Could you check a few things on this drawing? It's one solid part, dimensions in mm from its lowest x, y, z. A direction names the side the tool comes from. Give positions to 0.01 mm unless a question says otherwise; leave off trailing zeros. Loops run counter-clockwise (first coordinate to the right, second up) from the corner with the lowest first, then second, coordinate; pieces in that order, holes last. Notation, with made-up numbers: M -23,-17.75 L 28,-17.75 A30 cw 28,10.25 Z; hole C -36,72.5 d8. An arc over 180 degrees is marked long. Return JSON: item names as keys, results as strings. Group by question number.
1. If we section it at D-D (x = 144): Write out the boundary of the cut face in (y, z), plus the area to 3 significant figures.
2. Please list where these lines run through material, in increasing order: line 1 (X direction, y = 18.5, z = 7); line 2 (Y direction, x = 80.5, z = 52); line 3 (Z direction, x = 131, y = 30.5).
3. If we section it at B-B (y = 16.5): Write out the boundary of the cut face in (x, z) (1 decimal), plus the area to 3 significant figures.
4. For pin 1 (12 mm diameter, centred on x = 52.5, y = 52.5, fed in from -Z); pin 2 (4 mm diameter, centred on x = 97, y = 59.5, fed in from +Z); pin 3 (4 mm diameter, centred on x = 50.5, y = 47.5, fed in from -Z), each with a flat end and sliding along its axis, tell me the tip position at first contact or that it passes through.
5. For the marked faces 1, 2 and 3, which set-ups out of +Z, -Z, +X, -X, +Y, -Y let a thin tool reach every point of the face, with its end or its side?
6. If we section it at C-C (x = 47): Write out the boundary of the cut face in (y, z).
7. If we section it at A-A (z = 51.5): Write out the boundary of the cut face in (x, y), plus the area to 3 significant figures.
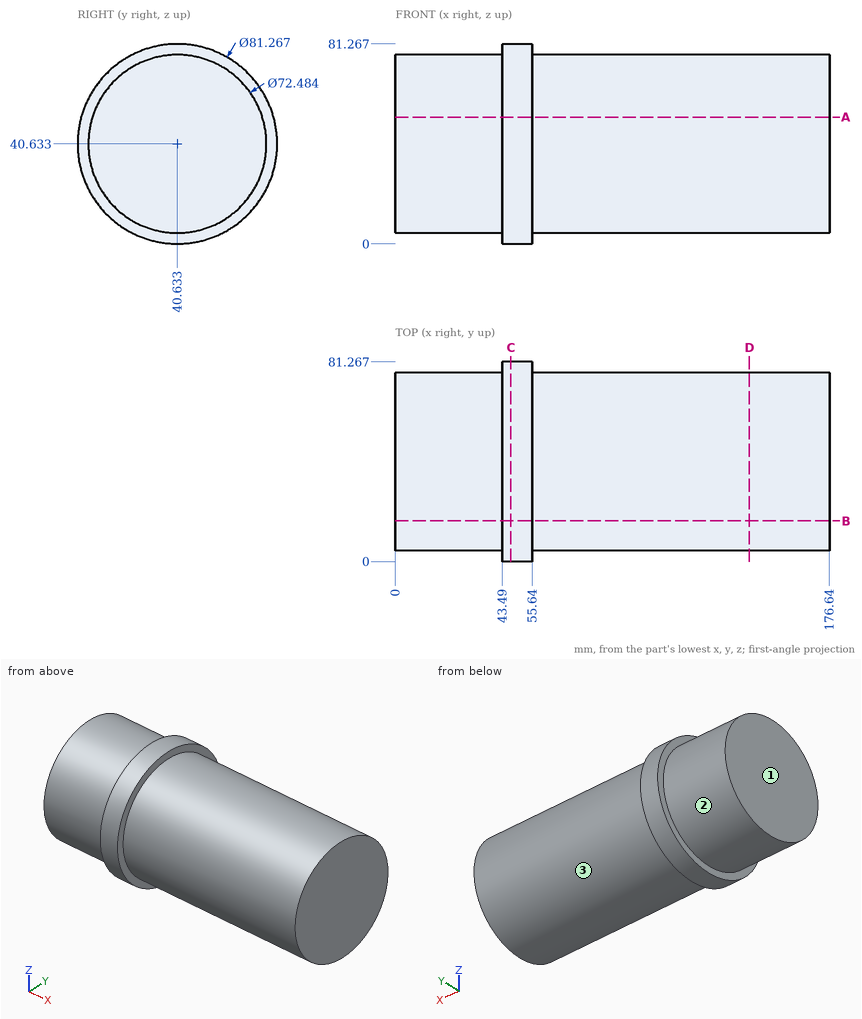
Answer:
{
 "1": {"outline": "C 40.63,40.63 d72.48", "area": "4,130 mm²"},
 "2": {"line 1": "x = 43.49 to 55.64", "line 2": "y = 6.22 to 75.05", "line 3": "z = 5.84 to 75.43"},
 "3": {"outline": "M 0,13.6 L 43.5,13.6 L 43.5,7.9 L 55.6,7.9 L 55.6,13.6 L 176.6,13.6 L 176.6,67.7 L 55.6,67.7 L 55.6,73.3 L 43.5,73.3 L 43.5,67.7 L 0,67.7 Z", "area": "9,690 mm²"},
 "4": {"pin 1": "stops at z = 0.43", "pin 2": "stops at z = 72.71", "pin 3": "stops at z = 0.29"},
 "5": {"face 1": "+Z, -Z, -X, +Y, -Y", "face 2": "-X", "face 3": "+X"},
 "6": {"outline": "C 40.63,40.63 d81.27"},
 "7": {"outline": "M 0,6.06 L 43.49,6.06 L 43.49,1.48 L 55.64,1.48 L 55.64,6.06 L 176.64,6.06 L 176.64,75.21 L 55.64,75.21 L 55.64,79.79 L 43.49,79.79 L 43.49,75.21 L 0,75.21 Z", "area": "12,300 mm²"}
}
